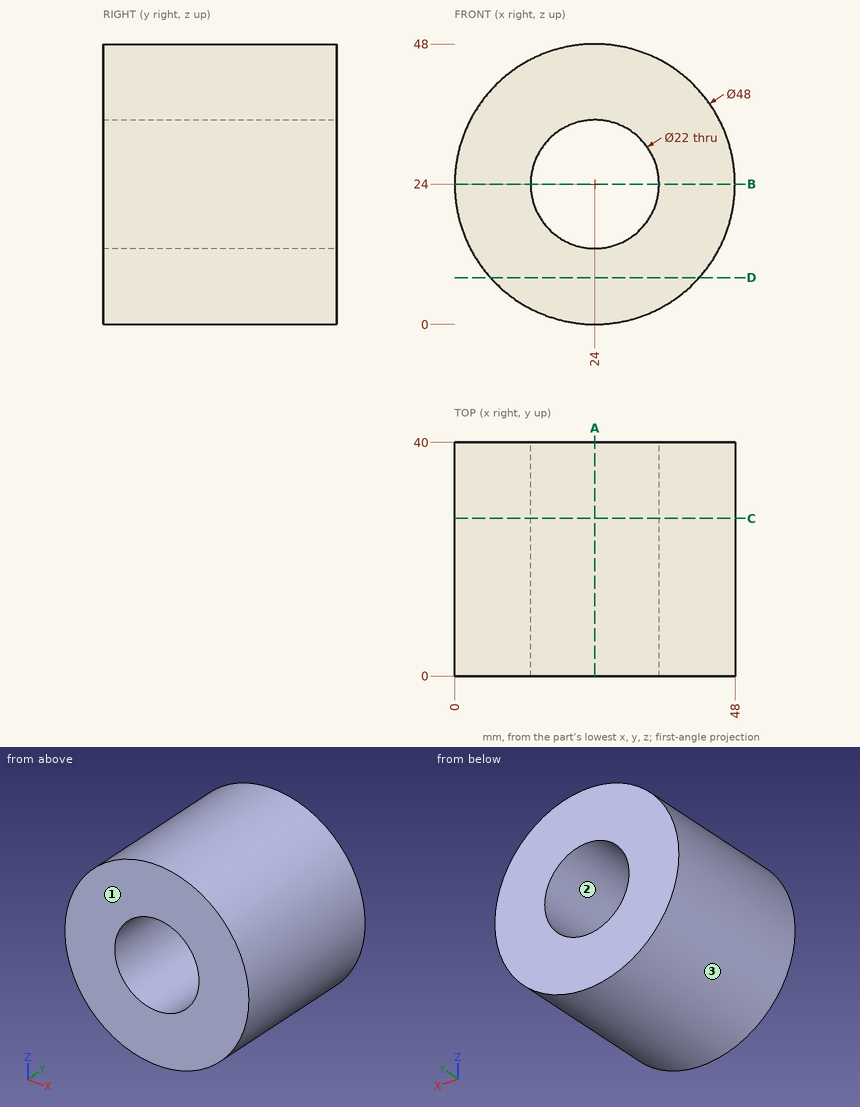
For this review, use the dimensioned drawing (mm, ordinates from the lowest corner) and the shaded views. Round coordinates to 2 decimals unless told otherwise and drop trailing zeros. Write each loop counter-clockwise with the first axis right and the second up, starting at its lowest first coordinate (ties: lowest second). Pieces come first, ordered by that corner, then holes. Notation, with made-up numbers: (17.25, 58) -> (31.25, 58) arc R13 cw to (31.25, 77) -> close; hole circle Ø1 at (77, 60). An arc over 180 degrees is marked (long way). Use one line per item in the form item = value.
Q1. The part is to be moulded in two halves that separate along Z. For the marked faces 1, 2 and 3, say which applies: released by +Z, released by -Z, zero draft, split by the parting line, or undercut.
Resolved:
face_1 = zero draft
face_2 = undercut
face_3 = split by the parting line
Q2. Consider section D-D (z = 8). State the section outline as (x, y) points.
Resolved:
outline = (6.11, 0) -> (41.89, 0) -> (41.89, 40) -> (6.11, 40) -> close
Q3. Clearance check with flat-ended pins moving along their axes: pin 1 Ø5 at (x, y) = (11.5, 27) entering from -Z; pin 2 Ø12 at (x, y) = (42.5, 13) entering from -Z; pin 3 Ø8 at (x, y) = (28, 8.5) entering from -Z. State where each tip first meets the part, or that it passes through.
Resolved:
pin_1 = 2.18
pin_2 = 3.51
pin_3 = 0
Q4. Consider section C-C (y = 27). State the section outline as (x, z) points.
Resolved:
outline = circle Ø48 at (24, 24); hole circle Ø22 at (24, 24)
Q5. Consider section B-B (z = 24). State the section outline as (x, y) points, then the cut area to 3 significant figures.
Resolved:
outline = (0, 0) -> (13, 0) -> (13, 40) -> (0, 40) -> close; (35, 0) -> (48, 0) -> (48, 40) -> (35, 40) -> close
area = 1,040 mm²
Q6. Consider section A-A (x = 24). State the section outline as (y, z) points.
Resolved:
outline = (0, 0) -> (40, 0) -> (40, 13) -> (0, 13) -> close; (0, 35) -> (40, 35) -> (40, 48) -> (0, 48) -> close
Q7. To check wall thickness, follow probe 1 along Z at (x, y) = (24, 23.5); probe 2 along X at (y, z) = (16, 21); probe 3 along Z at (x, y) = (34, 38.5). State the ranges of each line that lie inside material, in increasing order. Write a range as from..to.
Resolved:
probe_1 = 0..13, 35..48
probe_2 = 0.19..13.42, 34.58..47.81
probe_3 = 2.18..19.42, 28.58..45.82
